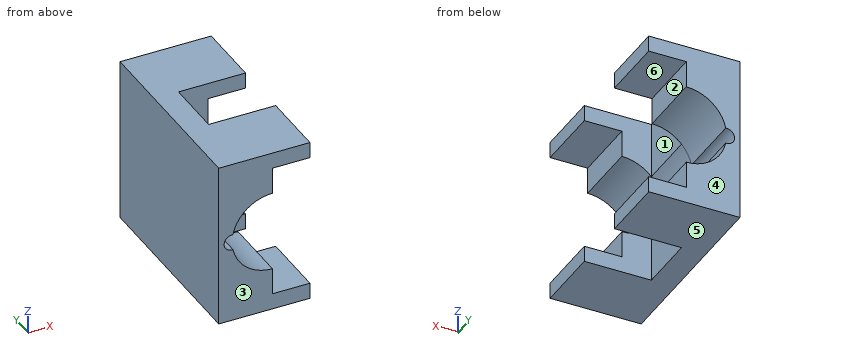
from build123d import *

# Parameters (mm, degrees)
BOSS_EXTRUDE1_DEPTH = 25
BOSS_EXTRUDE2_DEPTH = 22


with BuildPart() as part:
    # Sketch1 → Boss-Extrude1 (new body)
    with BuildSketch(Plane(origin=(0, 0, 0), x_dir=(1, 0, 0), z_dir=(0, 1, 0))):
        with BuildLine():
            Line((0, 25), (14, 25))
            Line((14, 25), (14, 31))
            Line((14, 31), (-20, 31))
            Line((-20, 31), (-20, -31))
            Line((-20, -31), (14, -31))
            Line((14, -31), (14, -25))
            Line((14, -25), (0, -25))
            Line((0, -25), (0, -15))
            ThreePointArc((0, -15), (-9.492775288, -11.614095631), (-14.7, -2.984962311))
            ThreePointArc((-14.7, -2.984962311), (-18, 0), (-14.7, 2.984962311))
            ThreePointArc((-14.7, 2.984962311), (-9.492775288, 11.614095631), (0, 15))
            Line((0, 15), (0, 25))
        make_face()
    boss_extrude1 = extrude(amount=BOSS_EXTRUDE1_DEPTH)

    # Sketch2 → Boss-Extrude2 (add)
    with BuildSketch(Plane(origin=(0, 25, 0), x_dir=(1, 0, 0), z_dir=(0, 1, 0))):
        with BuildLine():
            Line((-20, 31), (-20, -31))
            Line((-20, -31), (-11, -31))
            Line((-11, -31), (-11, -10.198039027))
            ThreePointArc((-11, -10.198039027), (-13.346520855, -6.846194642), (-14.7, -2.984962311))
            ThreePointArc((-14.7, -2.984962311), (-18, 0), (-14.7, 2.984962311))
            ThreePointArc((-14.7, 2.984962311), (-13.346520855, 6.846194642), (-11, 10.198039027))
            Line((-11, 10.198039027), (-11, 31))
            Line((-11, 31), (-20, 31))
        make_face()
    extrude(amount=BOSS_EXTRUDE2_DEPTH)

    # Mirror1: Boss-Extrude1 across plane
    add(boss_extrude1.mirror(Plane.ZX.offset(36)))


solid = part.part
Work out the finished part from the listing and answer in its coordinate system (mm). Face numbers are marked on the shaded views. A direction names the side the tool comes from. Give positions to 0.01 mm unless a question says otherwise; leave off trailing zeros. Order: outer loops, then holes, each group sorted by start corner. A loop starts at its lowest first (then second) coordinate and runs counter-clockwise, first axis right, second up. Notation, with made-up numbers: (80, 80.5) -> (131, 80.5) arc R24 ccw to (131, 115.5) -> close; hole circle Ø5 at (22.5, 85.5). An arc over 180 degrees is marked (long way). One line per item, written item: value.
Item 1: Determine the mould class of the marked faces 4, 5 and 6 for opening direction Z: released by +Z, released by -Z, zero draft, split by the parting line, or undercut.
Answer sheet:
face 4: zero draft
face 5: released by -Z
face 6: undercut
Item 2: Find section A-A, the plane x = 8.5. Give the vertices of the cut face in (y, z).
Answer sheet:
outline: (0, -31) -> (25, -31) -> (25, -25) -> (0, -25) -> close; (0, 25) -> (25, 25) -> (25, 31) -> (0, 31) -> close; (47, -31) -> (72, -31) -> (72, -25) -> (47, -25) -> close; (47, 25) -> (72, 25) -> (72, 31) -> (47, 31) -> close
Item 3: Flat-ended cylindrical pins translate along their axes: P1, Ø1.5, axis at y = 21, z = -5, coming from the +X side; P2, Ø3, axis at y = 65.5, z = -18.5, coming from the +X side; P3, Ø10.5, axis at x = 0.5, z = 19.5, coming from the -Y side; P4, Ø6, axis at y = 30.5, z = 17, coming from the +X side. Find the tip coordinate at first contact, or state that the pin passes through.
Answer sheet:
P1: x = -13.85
P2: x = 0
P3: y = 0
P4: x = -11
Item 4: Find section D-D, the plane x = -16. Give the vertices of the cut face in (y, z).
Answer sheet:
outline: (0, -31) -> (72, -31) -> (72, -2.83) -> (0, -2.83) -> close; (0, 2.83) -> (72, 2.83) -> (72, 31) -> (0, 31) -> close
Item 5: Find section C-C, the plane z = 27. Give the vertices of the cut face in (x, y), plus the area to 3 significant figures.
Answer sheet:
outline: (-20, 0) -> (14, 0) -> (14, 25) -> (-11, 25) -> (-11, 47) -> (14, 47) -> (14, 72) -> (-20, 72) -> close
area: 1,900 mm²
Item 6: A tool of negligible diameter and unlimited length cuts with its end or side. For the marked faces 1, 2 and 3, from which of +Z, -Z, +X, -X, +Y, -Y can it reach the whole face along a straight path? Write none if from no direction.
Answer sheet:
face 1: +Z, -Z, +X
face 2: +X, +Y, -Y
face 3: +Z, -Z, +X, -X, -Y
Item 7: Straight lines are drawn through the part: probe 1 along Z at (x, y) = (-15, 39); probe 2 along X at (y, z) = (7.5, -17); probe 3 along Z at (x, y) = (-2, 49). For each, find the intervals that lie inside material, in ascending order.
Answer sheet:
probe 1: -31 to -3, 3 to 31
probe 2: -20 to 0
probe 3: -31 to -14.87, 14.87 to 31
Item 8: Find section B-B, the plane y = 28. Give the vertices of the cut face in (x, z).
Answer sheet:
outline: (-20, -31) -> (-11, -31) -> (-11, -10.2) arc R15 cw to (-14.7, -2.98) arc R3 cw (long way) to (-14.7, 2.98) arc R15 cw to (-11, 10.2) -> (-11, 31) -> (-20, 31) -> close
